Geometry: final body of the model. Coordinates: model frame, mm. Give positions to 0.01 mm unless a question says otherwise; leave off trailing zeros. Loops run counter-clockwise (first coordinate to the right, second up) from the corner with the lowest first, then second, coordinate; pieces in that order, holes last.
from build123d import *

# Parameters (mm, degrees)
SKETCH1_R           = 6
BOSS_EXTRUDE1_DEPTH = 7.5
SKETCH3_R           = 6
CUT_EXTRUDE1_DEPTH  = 30.479866011
CIRPATTERN1_COUNT   = 4
SCALE1_SCALE        = 0.828947368


with BuildPart() as part:
    # Sketch1 → Boss-Extrude1 (new, symmetric)
    with BuildSketch(Plane.XY):
        Polygon((-12.75, 7.75), (-7.75, 12.75), (7.75, 12.75), (12.75, 7.75), (12.75, -7.75), (7.75, -12.75), (-7.75, -12.75), (-12.75, -7.75), align=None)
        Circle(SKETCH1_R, mode=Mode.SUBTRACT)
    extrude(amount=BOSS_EXTRUDE1_DEPTH, both=True)

    # Sketch3 → Cut-Extrude1 (cut, through all)
    with BuildSketch(Plane(origin=(0, 12.75, 0), x_dir=(1, 0, 0), z_dir=(0, 1, 0))):
        with Locations(Location((0, 0, 0), (0, 0, 270))):
            Circle(SKETCH3_R)
    cut_extrude1 = extrude(amount=-CUT_EXTRUDE1_DEPTH, mode=Mode.SUBTRACT)

    # CirPattern1: Cut-Extrude1 ×4 about axis
    cirpattern1_axis = Axis((0, 0, 7.5), (0, 0, -1))
    for i in range(1, CIRPATTERN1_COUNT):
        add(cut_extrude1.rotate(cirpattern1_axis, i * 360 / CIRPATTERN1_COUNT), mode=Mode.SUBTRACT)


with BuildPart() as part_1:
    # Scale1: scaled about (0, 0, 0)
    add(part.part.scale(SCALE1_SCALE))


solid = part_1.part
Item 1: Draft query along X for faces 1 (the face through (-3.666, 3.361, 5.148)), 2 (the face through (5, 2, 6.217)), 3 (the face through (-10.569, -2.95, 4.23)). Return one class per face: +X half, -X half, draft (parallel to the pull), parting line (faces both ways), or undercut.
Values follow:
face 1: undercut
face 2: draft
face 3: -X half
Item 2: Ray query, probe 1 along Z at (x, y) = (-5.5, 0); probe 2 along X at (y, z) = (-5.5, 0). Return the intervals inside material, ascending.
Values follow:
probe 1: z = -6.22 to -4.97, 4.97 to 6.22
probe 2: x = -10.57 to -4.97, 4.97 to 10.57
Item 3: Section query D-D on y = 4.25. Return loops of the section in (x, z), plus the area to 3 significant figures.
Values follow:
outline: (-10.57, -6.22) - (-2.58, -6.22) - (-2.58, -4.25) arc R4.97 cw to (-4.25, -2.58) - (-10.57, -2.58) - close; (-10.57, 2.58) - (-4.25, 2.58) arc R4.97 cw to (-2.58, 4.25) - (-2.58, 6.22) - (-10.57, 6.22) - close; (2.58, -6.22) - (10.57, -6.22) - (10.57, -2.58) - (4.25, -2.58) arc R4.97 cw to (2.58, -4.25) - close; (2.58, 4.25) arc R4.97 cw to (4.25, 2.58) - (10.57, 2.58) - (10.57, 6.22) - (2.58, 6.22) - close
area: 110 mm2
Item 4: Section query A-A on y = 0. Return loops of the section in (x, z), plus the area to 3 significant figures.
Values follow:
outline: (-10.57, -6.22) - (-4.97, -6.22) - (-4.97, -4.97) - (-10.57, -4.97) - close; (-10.57, 4.97) - (-4.97, 4.97) - (-4.97, 6.22) - (-10.57, 6.22) - close; (4.97, -6.22) - (10.57, -6.22) - (10.57, -4.97) - (4.97, -4.97) - close; (4.97, 4.97) - (10.57, 4.97) - (10.57, 6.22) - (4.97, 6.22) - close
area: 27.8 mm2
Item 5: Section query C-C on z = 0. Return loops of the section in (x, y).
Values follow:
outline: (-10.57, -6.42) - (-6.42, -10.57) - (-4.97, -10.57) - (-4.97, -4.97) - (-10.57, -4.97) - close; (-10.57, 4.97) - (-4.97, 4.97) - (-4.97, 10.57) - (-6.42, 10.57) - (-10.57, 6.42) - close; (4.97, -10.57) - (6.42, -10.57) - (10.57, -6.42) - (10.57, -4.97) - (4.97, -4.97) - close; (4.97, 4.97) - (10.57, 4.97) - (10.57, 6.42) - (6.42, 10.57) - (4.97, 10.57) - close
